from build123d import *

# Parameters (mm, degrees)
F1_DEPTH     = 3
F2_DEPTH     = 3
F4_DEPTH     = 4
F5_DEPTH     = 4
F6_T1_DEPTH  = 40.486982059
F6_T3_DEPTH  = 40.486982059
F6_T8_DEPTH  = 76.9380455506
F6_T13_DEPTH = 76.9380455506
F6_T18_DEPTH = 76.9380455506
F6_T23_DEPTH = 76.9380455506
F6_T28_DEPTH = 26.5734639037
F6_T35_DEPTH = 26.5734639037
F7_SIZE      = 3
F8_T4_DEPTH  = 125
F8_T10_DEPTH = 125
F8_T16_DEPTH = 125
F8_T22_DEPTH = 125
F9_DEPTH     = 5
F10_DEPTH    = 5
F11_SIZE     = 0.99999
F12_DEPTH    = 4
F13_DEPTH    = 4
F14_SIZE     = 3.99999


# Not quite as in the source:
# - a fillet or chamfer that OpenCascade refuses, or shapes differently, is made with other operations: its cross-section is extruded or revolved along the edge and cut away or added
# - a fillet or chamfer is up to 0.001 mm smaller than in the source, because OpenCascade refuses the exact size


with BuildPart() as f1:
    # F0 (on Right) → F1 (new body)
    with BuildSketch(Plane.YZ):
        Polygon((-3, 55), (-3, 0), (-3, -55), (3, -55), (3, 0), (3, 55), align=None)
    extrude(amount=F1_DEPTH)

    # F0 (on Right) → F2 (join)
    with BuildSketch(Plane.YZ):
        Polygon((-3, 55), (-3, 0), (-3, -55), (3, -55), (3, 0), (3, 55), align=None)
    extrude(amount=-F2_DEPTH)

    # F0 (on Right) → F4 (join)
    with BuildSketch(Plane.YZ):
        Polygon((-14.1003550962, 36.2719446421), (-3, 55), (3, 55), (14.1003550962, 36.2719446421), (20.8685267717, 55), (3, 108.4572896361), (0, 121.4577183127), (-3, 108.4572896361), (-20.8685267717, 55), align=None)
    extrude(amount=F4_DEPTH)

    # F3 (on face) + F0 (on Right) → F5 (join)
    with BuildSketch(Plane.YZ):
        Polygon((-7.805341389, 59.3111515045), (-3.0717977788, 55.1912151277), (3.0717977788, 55.1912151277), (7.805341389, 59.3111515045), (9.517685743, 63.5261535645), (11.2300300971, 67.7411556244), (0, 96.2772667408), (-11.2300300971, 67.7411556244), (-9.517685743, 63.5261535645), align=None)
        Polygon((9.517685743, 63.5261535645), (7.805341389, 59.3111515045), (11.814879576, 47.7191654262), (14.9534028023, 55.4447621107), align=None)
    with BuildSketch(Plane.YZ):
        Polygon((-14.1003550962, 36.2719446421), (-3, 55), (3, 55), (14.1003550962, 36.2719446421), (20.8685267717, 55), (3, 108.4572896361), (0, 121.4577183127), (-3, 108.4572896361), (-20.8685267717, 55), align=None)
    extrude(amount=-F5_DEPTH)

    # F6: chamfer of 4 on 10 edges, made by hand

    # F6_s2 → F6_t1 (cut)
    with BuildSketch(Plane(origin=(0, -23.4873916457, 64.9914322573), x_dir=(1, 0, 0), z_dir=(0, 0.3398782487, -0.9404694445))):
        Polygon((0, 0.932908104), (4, -3.067091896), (4, 0.932908104), align=None)
        Polygon((-4, -3.067091896), (0, 0.932908104), (-4, 0.932908104), align=None)
    extrude(amount=F6_T1_DEPTH, mode=Mode.SUBTRACT)

    # F6_s4 → F6_t3 (cut)
    with BuildSketch(Plane(origin=(0, 9.7267470895, 26.9146627299), x_dir=(1, 0, 0), z_dir=(0, 0.3398782487, 0.9404694445))):
        Polygon((4, -3.067091896), (0, 0.932908104), (4, 0.932908104), align=None)
        Polygon((-4, -3.067091896), (0, 0.932908104), (-4, 0.932908104), align=None)
    extrude(amount=F6_T3_DEPTH, mode=Mode.SUBTRACT)


with BuildPart() as f6_tool6:
    # F6_s7 → F6_t8 (new body)
    with BuildSketch(Plane(origin=(0, -11.1782341891, 33.4419345425), x_dir=(1, 0, 0), z_dir=(0, -0.3170169324, 0.9484198778))):
        Polygon((4, 33.2280568939), (0, 37.2280568939), (4, 37.2280568939), align=None)
    extrude(amount=F6_T8_DEPTH)

    split(bisect_by=Plane(origin=(0, 26.6107337931, 6.1407360761), x_dir=(1, 0, 0), z_dir=(0, 0.9743928202, 0.224852467)), keep=Keep.TOP)


with BuildPart() as f1_1:
    add(f1.part)

    # F6_t5: cut F6_tool6
    add(f6_tool6.part, mode=Mode.SUBTRACT)


with BuildPart() as f6_tool11:
    # F6_s12 → F6_t13 (new body)
    with BuildSketch(Plane(origin=(0, 35.5688973771, 106.4115062996), x_dir=(1, 0, 0), z_dir=(0, -0.3170169324, -0.9484198778))):
        Polygon((4, 33.2280568939), (0, 37.2280568939), (4, 37.2280568939), align=None)
    extrude(amount=F6_T13_DEPTH)

    split(bisect_by=Plane(origin=(0, -26.6107337931, 6.1407360761), x_dir=(1, 0, 0), z_dir=(0, -0.9743928202, 0.224852467)), keep=Keep.TOP)


with BuildPart() as f1_2:
    add(f1_1.part)

    # F6_t10: cut F6_tool11
    add(f6_tool11.part, mode=Mode.SUBTRACT)


with BuildPart() as f6_tool16:
    # F6_s17 → F6_t18 (new body)
    with BuildSketch(Plane(origin=(0, 35.5688973771, 106.4115062996), x_dir=(1, 0, 0), z_dir=(0, -0.3170169324, -0.9484198778))):
        Polygon((-4, 33.2280568939), (0, 37.2280568939), (-4, 37.2280568939), align=None)
    extrude(amount=F6_T18_DEPTH)

    split(bisect_by=Plane(origin=(0, -26.6107337931, 6.1407360761), x_dir=(1, 0, 0), z_dir=(0, -0.9743928202, 0.224852467)), keep=Keep.TOP)


with BuildPart() as f1_3:
    add(f1_2.part)

    # F6_t15: cut F6_tool16
    add(f6_tool16.part, mode=Mode.SUBTRACT)


with BuildPart() as f6_tool21:
    # F6_s22 → F6_t23 (new body)
    with BuildSketch(Plane(origin=(0, -11.1782341891, 33.4419345425), x_dir=(1, 0, 0), z_dir=(0, -0.3170169324, 0.9484198778))):
        Polygon((-4, 33.2280568939), (0, 37.2280568939), (-4, 37.2280568939), align=None)
    extrude(amount=F6_T23_DEPTH)

    split(bisect_by=Plane(origin=(0, 26.6107337931, 6.1407360761), x_dir=(1, 0, 0), z_dir=(0, 0.9743928202, 0.224852467)), keep=Keep.TOP)


with BuildPart() as f1_4:
    add(f1_3.part)

    # F6_t20: cut F6_tool21
    add(f6_tool21.part, mode=Mode.SUBTRACT)


with BuildPart() as f6_tool26:
    # F6_s27 → F6_t28 (new body)
    with BuildSketch(Plane.XZ.offset(13.2867319519)):
        Polygon((0, 55), (-4, 59), (-4, 55), align=None)
    extrude(amount=-F6_T28_DEPTH)

    split(bisect_by=Plane.YZ.offset(-3), keep=Keep.BOTTOM)

    split(bisect_by=Plane(origin=(0, 26.3442442024, 15.6145664778), x_dir=(1, 0, 0), z_dir=(0, -0.8602462388, -0.5098788176)), keep=Keep.TOP)

    split(bisect_by=Plane(origin=(0, -26.3442442024, 15.6145664778), x_dir=(1, 0, 0), z_dir=(0, 0.8602462388, -0.5098788176)), keep=Keep.TOP)


with BuildPart() as f1_5:
    add(f1_4.part)

    # F6_t25: cut F6_tool26
    add(f6_tool26.part, mode=Mode.SUBTRACT)


with BuildPart() as f6_tool33:
    # F6_s34 → F6_t35 (new body)
    with BuildSketch(Plane.XZ.offset(13.2867319519)):
        Polygon((4, 59), (0, 55), (4, 55), align=None)
    extrude(amount=-F6_T35_DEPTH)

    split(bisect_by=Plane.YZ.offset(3), keep=Keep.TOP)

    split(bisect_by=Plane(origin=(0, 26.3442442024, 15.6145664778), x_dir=(1, 0, 0), z_dir=(0, -0.8602462388, -0.5098788176)), keep=Keep.TOP)

    split(bisect_by=Plane(origin=(0, -26.3442442024, 15.6145664778), x_dir=(1, 0, 0), z_dir=(0, 0.8602462388, -0.5098788176)), keep=Keep.TOP)


with BuildPart() as f1_6:
    add(f1_5.part)

    # F6_t32: cut F6_tool33
    add(f6_tool33.part, mode=Mode.SUBTRACT)

    # F7
    f7_edges = [f1_6.edges().sort_by_distance(p)[0] for p in [
        (4, 6.201839, 94.582196),
        (4, -6.201839, 94.582196),
        (-4, -6.201839, 94.582196),
        (-4, 6.201839, 94.582196),
    ]]
    chamfer(f7_edges, length=F7_SIZE)

    # F8: fillet of radius 3 on 4 edges, made by hand


with BuildPart() as f8_tool2:
    # F8_s3 → F8_t4 (new body)
    with BuildSketch(Plane.XY.offset(62.5)):
        with BuildLine():
            ThreePointArc((0, -3), (-2.1213203436, -2.1213203436), (-3, 0))
            Line((-3, 0), (-3, -3))
            Line((-3, -3), (0, -3))
        make_face()
    extrude(amount=-F8_T4_DEPTH)

    split(bisect_by=Plane(origin=(0, -26.3442442024, 15.6145664778), x_dir=(1, 0, 0), z_dir=(0, 0.8602462388, -0.5098788176)), keep=Keep.TOP)

    split(bisect_by=Plane(origin=(27.5, 0, 27.5), x_dir=(0, 1, 0), z_dir=(-0.7071067812, 0, -0.7071067812)), keep=Keep.TOP)


with BuildPart() as f1_7:
    add(f1_6.part)

    # F8_t1: cut F8_tool2
    add(f8_tool2.part, mode=Mode.SUBTRACT)


with BuildPart() as f8_tool8:
    # F8_s9 → F8_t10 (new body)
    with BuildSketch(Plane.XY.offset(-62.5)):
        with BuildLine():
            ThreePointArc((-3, 0), (-2.1213203436, 2.1213203436), (0, 3))
            Line((0, 3), (-3, 3))
            Line((-3, 3), (-3, 0))
        make_face()
    extrude(amount=F8_T10_DEPTH)

    split(bisect_by=Plane(origin=(27.5, 0, 27.5), x_dir=(0, 1, 0), z_dir=(-0.7071067812, 0, -0.7071067812)), keep=Keep.TOP)

    split(bisect_by=Plane(origin=(0, 26.3442442024, 15.6145664778), x_dir=(1, 0, 0), z_dir=(0, -0.8602462388, -0.5098788176)), keep=Keep.TOP)


with BuildPart() as f1_8:
    add(f1_7.part)

    # F8_t7: cut F8_tool8
    add(f8_tool8.part, mode=Mode.SUBTRACT)


with BuildPart() as f8_tool14:
    # F8_s15 → F8_t16 (new body)
    with BuildSketch(Plane.XY.offset(62.5)):
        with BuildLine():
            ThreePointArc((3, 0), (2.1213203436, 2.1213203436), (0, 3))
            Line((0, 3), (3, 3))
            Line((3, 3), (3, 0))
        make_face()
    extrude(amount=-F8_T16_DEPTH)

    split(bisect_by=Plane(origin=(0, 26.3442442024, 15.6145664778), x_dir=(1, 0, 0), z_dir=(0, -0.8602462388, -0.5098788176)), keep=Keep.TOP)

    split(bisect_by=Plane(origin=(-27.5, 0, 27.5), x_dir=(0, 1, 0), z_dir=(0.7071067812, 0, -0.7071067812)), keep=Keep.TOP)


with BuildPart() as f1_9:
    add(f1_8.part)

    # F8_t13: cut F8_tool14
    add(f8_tool14.part, mode=Mode.SUBTRACT)


with BuildPart() as f8_tool20:
    # F8_s21 → F8_t22 (new body)
    with BuildSketch(Plane.XY.offset(-62.5)):
        with BuildLine():
            ThreePointArc((3, 0), (2.1213203436, -2.1213203436), (0, -3))
            Line((0, -3), (3, -3))
            Line((3, -3), (3, 0))
        make_face()
    extrude(amount=F8_T22_DEPTH)

    split(bisect_by=Plane(origin=(0, -26.3442442024, 15.6145664778), x_dir=(1, 0, 0), z_dir=(0, 0.8602462388, -0.5098788176)), keep=Keep.TOP)

    split(bisect_by=Plane(origin=(-27.5, 0, 27.5), x_dir=(0, 1, 0), z_dir=(0.7071067812, 0, -0.7071067812)), keep=Keep.TOP)


with BuildPart() as f1_10:
    add(f1_9.part)

    # F8_t19: cut F8_tool20
    add(f8_tool20.part, mode=Mode.SUBTRACT)

    # F3 (on face) → F9 (join)
    with BuildSketch(Plane.YZ):
        Polygon((-7.805341389, 59.3111515045), (-3.0717977788, 55.1912151277), (3.0717977788, 55.1912151277), (7.805341389, 59.3111515045), (9.517685743, 63.5261535645), (11.2300300971, 67.7411556244), (0, 96.2772667408), (-11.2300300971, 67.7411556244), (-9.517685743, 63.5261535645), align=None)
        Polygon((-11.814879576, 47.7191654262), (-7.805341389, 59.3111515045), (-9.517685743, 63.5261535645), (-14.9534028023, 55.4447621107), align=None)
        Polygon((9.517685743, 63.5261535645), (7.805341389, 59.3111515045), (11.814879576, 47.7191654262), (14.9534028023, 55.4447621107), align=None)
    extrude(amount=F9_DEPTH)

    # F3 (on face) → F10 (join)
    with BuildSketch(Plane.YZ):
        Polygon((-7.805341389, 59.3111515045), (-3.0717977788, 55.1912151277), (3.0717977788, 55.1912151277), (7.805341389, 59.3111515045), (9.517685743, 63.5261535645), (11.2300300971, 67.7411556244), (0, 96.2772667408), (-11.2300300971, 67.7411556244), (-9.517685743, 63.5261535645), align=None)
        Polygon((-11.814879576, 47.7191654262), (-7.805341389, 59.3111515045), (-9.517685743, 63.5261535645), (-14.9534028023, 55.4447621107), align=None)
        Polygon((9.517685743, 63.5261535645), (7.805341389, 59.3111515045), (11.814879576, 47.7191654262), (14.9534028023, 55.4447621107), align=None)
    extrude(amount=-F10_DEPTH)

    # F11 (size 1 in the source; OpenCascade refuses exactly that, so slightly less here)
    f11_edges = [f1_10.edges().sort_by_distance(p)[0] for p in [
        (5, -5.43857, 57.251183),
        (5, 0, 55.191215),
        (5, 5.43857, 57.251183),
        (5, 9.81011, 53.515158),
        (5, 13.384141, 51.581964),
        (5, 12.235544, 59.485458),
        (5, 10.373858, 65.633655),
        (5, 5.615015, 82.009211),
        (5, -5.615015, 82.009211),
        (5, -10.373858, 65.633655),
        (5, -12.235544, 59.485458),
        (5, -13.384141, 51.581964),
        (5, -9.81011, 53.515158),
        (-5, -5.615015, 82.009211),
        (-5, -5.43857, 57.251183),
        (-5, 0, 55.191215),
        (-5, 5.43857, 57.251183),
        (-5, 9.81011, 53.515158),
        (-5, 13.384141, 51.581964),
        (-5, 12.235544, 59.485458),
        (-5, 10.373858, 65.633655),
        (-5, 5.615015, 82.009211),
        (-5, -10.373858, 65.633655),
        (-5, -12.235544, 59.485458),
        (-5, -13.384141, 51.581964),
        (-5, -9.81011, 53.515158),
    ]]
    chamfer(f11_edges, length=F11_SIZE)

    # F0 (on Right) → F12 (join)
    with BuildSketch(Plane.YZ):
        Polygon((3, -55), (-3, -55), (-8.9030144736, -52.6038594544), (0, -77.3145779967), (8.9030144736, -52.6038594544), align=None)
    extrude(amount=F12_DEPTH)

    # F0 (on Right) → F13 (join)
    with BuildSketch(Plane.YZ):
        Polygon((3, -55), (-3, -55), (-8.9030144736, -52.6038594544), (0, -77.3145779967), (8.9030144736, -52.6038594544), align=None)
    extrude(amount=-F13_DEPTH)

    # F14 (size 4 in the source; OpenCascade refuses exactly that, so slightly less here)
    f14_edges = [f1_10.edges().sort_by_distance(p)[0] for p in [
        (-4, -4.451507, -64.959219),
        (-4, 4.451507, -64.959219),
        (4, -4.451507, -64.959219),
        (4, 4.451507, -64.959219),
    ]]
    chamfer(f14_edges, length=F14_SIZE)


solid = f1_10.part
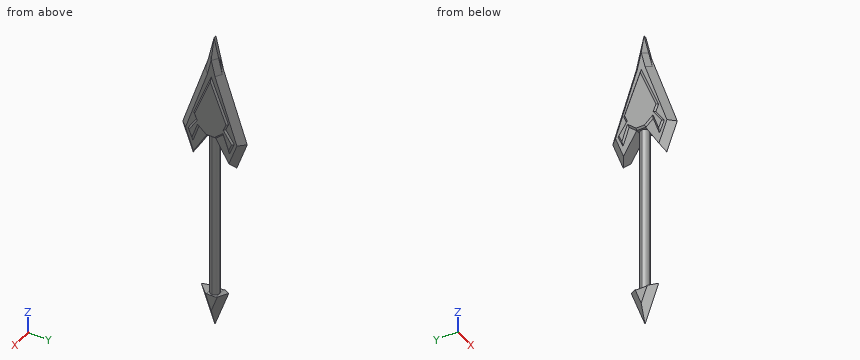
Here's how the part is built. I have some questions about the finished solid (model axes, mm). Coordinates: 2 decimals unless noted, no trailing zeros. Order: outer loops, then holes, each group sorted by start corner. A loop starts at its lowest first (then second) coordinate and runs counter-clockwise, first axis right, second up. Notation, with made-up numbers: (10.25, 1) -> (48.25, 1) arc R18 cw to (48.25, 28) -> close; hole circle Ø9 at (53.5, 82). An arc over 180 degrees is marked (long way). Answer in a Markdown table with one row per item.
(1) I want a section at B-B on z = 29. List the corners of the cut face in (x, y) for me.
Answer key:
| item | result |
|---|---|
| outline | circle Ø6 at (0, 0) |
(2) Please list where these lines run through material, in increasing order: probe 1 along Y at (x, z) = (-1.25, -14.5); probe 2 along Y at (x, z) = (1.5, 87.5); probe 3 along X at (y, z) = (-2, -41).
Answer key:
| item | result |
|---|---|
| probe 1 | -2.73 to 2.73 |
| probe 2 | -8.42 to 8.42 |
| probe 3 | -2.24 to 2.24 |
(3) I want a section at C-C on y = 18.5. List the corners of the cut face in (x, z) for me.
Answer key:
| item | result |
|---|---|
| outline | (-2.24, 55.03) -> (0, 48.45) -> (2.24, 55.03) -> (0, 62.09) -> close |
(4) Will these pins go through, and if not, where does the flat tip stop? pin 1 Ø8.5 at (y, z) = (-0.5, -58.5) entering from -X; pin 2 Ø6 at (x, y) = (1, 13) entering from -Z; pin 3 Ø4 at (y, z) = (-3, 18) entering from +X; pin 4 Ø4.5 at (x, y) = (-2, -0.5) entering from +Z.
Answer key:
| item | result |
|---|---|
| pin 1 | x = -4 |
| pin 2 | z = 36.27 |
| pin 3 | x = 2.83 |
| pin 4 | z = 121.46 |
